Can you work these out from the model? Positions are in its coordinate system, mm. A direction names the side the tool comes from. Give positions to 0.01 mm unless a question says otherwise; leave off trailing zeros. Order: outer loops, then holes, each group sorted by start corner. A loop starts at its lowest first (then second) coordinate and runs counter-clockwise, first axis right, second up.
Autodesk Inventor part; units mm, degrees
ref_plane "YZ Plane" through (0, 0, 0) normal (1, 0, 0) x (0, 1, 0)
ref_plane "XZ Plane" through (0, 0, 0) normal (0, 1, 0) x (-1, 0, 0)
ref_plane "XY Plane" through (0, 0, 0) normal (0, 0, 1) x (1, 0, 0)
sketch "Sketch1" plane through (0, 0, 0) normal (0, 0, 1) x (1, 0, 0)
  circle A0 centre (0, 0) radius 207.9625
  line L0 (-215.7457, 231.7761) -> (224.1521, 231.7761) construction
  line L1 (224.1521, 231.7761) -> (224.1521, -258.7625) construction
  line L2 (224.1521, -258.7625) -> (-207.6479, -258.7625) construction
  line L3 (0, 0) -> (294.0459, 0) construction
  line L4 (294.0459, 0) -> (62.2698, 231.7761) construction
  line L5 (294.0459, 0) -> (621.8269, 0) construction
  line L6 (-129.4556, -162.7564) -> (-480.3051, -162.7564) construction
  line L7 (-480.3051, -162.7564) -> (-480.3051, 0) construction
  line L8 (-480.3051, 0) -> (-129.4556, 0) construction
  line L9 (-129.4556, 0) -> (-129.4556, -162.7564) construction
  line L10 (62.2698, 231.7761) -> (294.0459, 0) construction
  line L11 (294.0459, 0) -> (599.7721, 305.7262)
  line L12 (599.7721, 305.7262) -> (367.996, 537.5023)
  line L13 (367.996, 537.5023) -> (62.2698, 231.7761)
  line L14 (-207.6479, -162.7564) -> (-207.6479, -258.7625)
  line L15 (-207.6479, -258.7625) -> (224.1521, -258.7625)
  line L16 (224.1521, -258.7625) -> (224.1521, 69.8938)
  line L17 (224.1521, 69.8938) -> (149.9298, 144.1161)
  line L18 (-207.6479, -162.7564) -> (-129.4556, -162.7564)
  line L19 (-207.6479, -258.7625) -> (-207.6479, -162.7564) construction
  line L20 (-215.7457, 0) -> (-215.7457, 231.7761) construction
  line L21 (0, -207.9625) -> (0, -258.7625)
  point P0 (-207.9625, 0)
  dimension "d0" = 415.925
  dimension "d3" = 135
  dimension "d6" = 431.8
  dimension "d7" = 50.8
extrude "Extrusion1" add sketch "Sketch1" along normal blind 50.8 contours A0 L17 L16 L15 L21 | L21 L15 L14 L18 A0
properties part number "main prototype"
1) Suppose I cut it at D-D (y = 0). Please give me the cut outline in (x, z).
2) Which directions (+Z, -Z, +X, -X, +Y, -Y) give clear straight access to the entire face, cutting with the end or side of a thin tool? Please do faces 5 (the face through (55, -206, 0)), 6 (the face through (-169, -162.756, 25)).
3) We'd pull the mould along X, two halves only. Please class faces 1 (the face through (187.561, 106.485, 25.044)), 2 (the face through (-207.648, -210, 25)), 3 (the face through (156.691, -136.734, 25.044)), 4 (the face through (5, -258.762, 25)): +X half, -X half, draft (parallel to the pull), parting line (faces both ways), or undercut.
4) Suppose I cut it at B-B (x = 0). Please give me the cut outline in (y, z), and give its area (3 significant figures).
5) I'm going to push flat-ended pins straight in: pin 1 Ø5 at (y, z) = (-119, 7.5) entering from -X; pin 2 Ø6 at (x, z) = (144, 34.5) entering from +Y; pin 3 Ø1 at (x, z) = (-90, 25.5) entering from +Y. Where does each tip first touch, or does it pass through?
6) Suppose I cut it at A-A (y = -190). Please give me the cut outline in (x, z).
7) Suppose I cut it at C-C (z = 26). Please give me the cut outline in (x, y) (1 decimal), and give its area (3 significant figures).
8) If I drill on line 1 (Y direction, x = 1, z = 5); line 2 (Y direction, x = -170.5, z = 30); line 3 (X direction, y = -177.5, z = 15), over which ranges is the centre line in solid material (lowest first)?
Results:
1. outline: (207.96, 0) - (224.15, 0) - (224.15, 50.8) - (207.96, 50.8) - close
2. face 5: -Z, +X, -X, +Y, -Y
2. face 6: +Z, -Z, -X, +Y
3. face 1: +X half
3. face 2: -X half
3. face 3: undercut
3. face 4: draft
4. outline: (-258.76, 0) - (-207.96, 0) - (-207.96, 50.8) - (-258.76, 50.8) - close
4. area: 2,580 mm2
5. pin 1: stops at x = 168.78
5. pin 2: stops at y = -147.1
5. pin 3: stops at y = -187.24
6. outline: (-207.65, 0) - (-84.55, 0) - (-84.55, 50.8) - (-207.65, 50.8) - close; (84.55, 0) - (224.15, 0) - (224.15, 50.8) - (84.55, 50.8) - close
7. outline: (-207.6, -258.8) - (224.2, -258.8) - (224.2, 69.9) - (149.9, 144.1) arc R208 cw to (-129.5, -162.8) - (-207.6, -162.8) - close
7. area: 42,200 mm2
8. line 1: y = -258.76 to -207.96
8. line 2: y = -258.76 to -162.76
8. line 3: x = -207.65 to -108.36, 108.36 to 224.15
